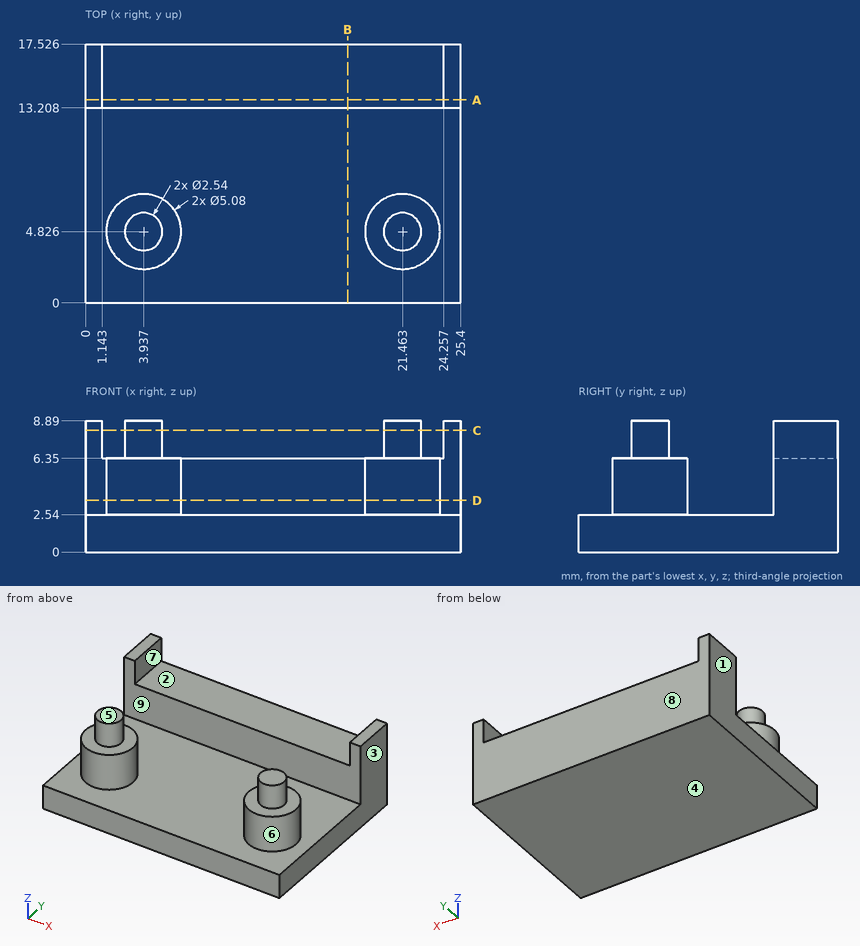
For this review, use the dimensioned drawing (mm, ordinates from the lowest corner) and the shaded views. A direction names the side the tool comes from. Round coordinates to 2 decimals unless told otherwise and drop trailing zeros. Write each loop counter-clockwise with the first axis right and the second up, starting at its lowest first coordinate (ties: lowest second). Pieces come first, ordered by that corner, then holes. Notation, with made-up numbers: M -21,23 L 23,23 A4 cw 23,30 Z; hole C 5,-37 d1. An arc over 180 degrees is marked long. Use CSV: the item, a comma, the result in double quotes. Start each with the question number.
(1) The part is to be moulded in two halves that separate along X. For the marked faces 1, 2, 3 and 4, say which applies: +X half, -X half, draft (parallel to the pull), parting line (faces both ways), or undercut.
(2) Tool access review of the marked faces 5, 6, 7, 8 and 9: name each direction out of +Z, -Z, +X, -X, +Y, -Y from which nothing blocks a thin tool from reaching the whole face with its end or side.
(3) For line 1 along X through (y, z) = (15.75, 6.75); line 2 along Z through (x, y) = (19, 7.75); line 3 along Z through (x, y) = (9.75, 15.5), list the stretches that pass through material, from the lowest coordinate up.
(4) Clearance check with flat-ended pins moving along their axes: P1, Ø4, axis at x = 12.5, y = 8.5, coming from the +Z side; P2, Ø2.5, axis at x = 2.5, y = 4.5, coming from the +Z side; P3, Ø5, axis at x = 18.5, z = 5.5, coming from the -Y side; P4, Ø2, axis at x = 13, y = 16.5, coming from the +Z side. State where each tip first meets the part, or that it passes through.
(5) We need section A-A, the plane y = 13.75. State the section outline as (x, z) points, then the cut area to 3 significant figures.
(6) We need section C-C, the plane z = 8.25. State the section outline as (x, y) points.
(7) We need section D-D, the plane z = 3.5. State the section outline as (x, y) points.
(8) We need section B-B, the plane x = 17.75. State the section outline as (y, z) points, then the cut area to 3 significant figures.
Findings:
1,face 1,"-X half"
1,face 2,"undercut"
1,face 3,"+X half"
1,face 4,"draft"
2,face 5,"+Z, +X, -X, +Y, -Y"
2,face 6,"+Z"
2,face 7,"+Z, +Y, -Y"
2,face 8,"+Z, -Z, +X, -X, +Y"
2,face 9,"+Z, +X, -X"
3,line 1,"0 to 1.14, 24.26 to 25.4"
3,line 2,"0 to 2.54"
3,line 3,"0 to 6.35"
4,P1,"z = 2.54"
4,P2,"z = 8.89"
4,P3,"y = 2.33"
4,P4,"z = 6.35"
5,outline,"M 0,0 L 25.4,0 L 25.4,8.89 L 24.26,8.89 L 24.26,6.35 L 1.14,6.35 L 1.14,8.89 L 0,8.89 Z"
5,area,"167 mm^2"
6,outline,"M 0,13.21 L 1.14,13.21 L 1.14,17.53 L 0,17.53 Z; C 3.94,4.83 d2.54; C 21.46,4.83 d2.54; M 24.26,13.21 L 25.4,13.21 L 25.4,17.53 L 24.26,17.53 Z"
7,outline,"M 0,13.21 L 25.4,13.21 L 25.4,17.53 L 0,17.53 Z; C 3.94,4.83 d5.08; C 21.46,4.83 d5.08"
8,outline,"M 0,0 L 17.53,0 L 17.53,6.35 L 13.21,6.35 L 13.21,2.54 L 0,2.54 Z"
8,area,"61.0 mm^2"
